Design review of the part built by this model. Coordinates are the model's own, in mm. A direction names the side the tool comes from. Coordinates: 2 decimals unless noted, no trailing zeros. Loops run counter-clockwise (first coordinate to the right, second up) from the corner with the lowest first, then second, coordinate; pieces in that order, holes last.
Q1. Draft analysis for pull direction Z (two halves, no side actions). For faces 6 (the face through (20.32, 58, 19)), 7 (the face through (0, -8, 38.1)), 8 (the face through (0, 58, 19.095)), 9 (the face through (6.846, 58, 23)), state which applies: released by +Z, released by -Z, zero draft, split by the parting line, or undercut.
Q2. Wall thickness on probe 1 along Y at (x, z) = (26.5, 2); probe 2 along X at (y, z) = (-6, 19.5); probe 3 along X at (y, z) = (19, 4.5): over which ranges is each line inside the solid? List them lowest first.
Q3. Add section B-B on x = 0. Give the number of separate pieces and of enclosed holes in the cut face, and give its area (3 significant figures).
Q4. Machinability: for faces 1 (the face through (0, -15.24, 28)), 2 (the face through (-0.674, -58.015, 27.798)), 3 (the face through (-7.733, 22, 6)), 4 (the face through (0, 66.04, 28)), 5 (the face through (20.32, -8, 19)), which of the approach directions +Z, -Z, +X, -X, +Y, -Y give a long, thin tool a straight path to every point of the face, cutting with its end or side? Answer none if there is none.
Q5. Add section A-A on y = 21.5. Give the boundary of the cut face in (x, z), and give its area (3 significant figures).
Q6. For P1, Ø4.5, axis at y = -9, z = 23, coming from the +X side; P2, Ø6, axis at y = 67.5, z = 21.5, coming from the -X side; P3, Ø7.5, axis at x = 3, z = 28.5, coming from the -Y side; P4, Ø14, axis at y = 57.5, z = 18.5, coming from the -X side, all flat-tipped, find the tip position at first contact; note any pin that passes through.
Q7. Add section C-C on z = 33.5. Give the boundary of the cut face in (x, y), and give its area (3 significant figures).
```python
from build123d import *

# Parameters (mm, degrees)
F1_DEPTH     = 12.7
F3_DEPTH     = 25.4
F4_R         = 12.7
F5_R         = 12.7
F6_R         = 12.7
F8_DEPTH     = 104.141
F9_W         = 26.8278098665
F9_H         = 37.2433126904
F10_DEPTH    = 12.701
F11_R        = 5.08
F12_R        = 12.1917967362
F12_R_2      = 5.1797647995
F13_DEPTH    = 5.08
F14_DEPTH    = 25.4
F15_SIZE     = 5.07999
F17_DEPTH    = 25.4
F18_R        = 5.08
F19_DEPTH    = 12.701
F21_DEPTH    = 12.701
F22_T1_DEPTH = 12.7
F23_R        = 2.794


# Not quite as in the source:
# - a fillet or chamfer that OpenCascade refuses, or shapes differently, is made with other operations: its cross-section is extruded or revolved along the edge and cut away or added
# - a fillet or chamfer is up to 0.001 mm smaller than in the source, because OpenCascade refuses the exact size
# - a feature names something its author has since deleted; it is built from what else it names


with BuildPart() as f1:
    # F0 (on Top) → F1 (new body)
    with BuildSketch(Plane.XY):
        Polygon((-50.8, 88.9), (-50.8, 0), (-50.8, -88.9), (0, -88.9), (50.8, -88.9), (50.8, 0), (50.8, 88.9), (0, 88.9), align=None)
    extrude(amount=F1_DEPTH)

    # F2 (on face) → F3 (join)
    with BuildSketch(Plane.XY.offset(12.7)):
        Polygon((20.32, 66.04), (0, 66.04), (-20.32, 66.04), (-20.32, 50.8), (0, 50.8), (20.32, 50.8), align=None)
        Polygon((0, 0), (-19.5459036618, 0), (-19.5459036618, -15.24), (0, -15.24), (20.32, -15.24), (20.32, 0), align=None)
    extrude(amount=F3_DEPTH)

    # F4
    f4_edges = [f1.edges().sort_by_distance(p)[0] for p in [
        (20.32, -7.62, 38.1),
        (-19.545904, -7.62, 38.1),
    ]]
    fillet(f4_edges, radius=F4_R)

    # F5
    f5_edges = [f1.edges().sort_by_distance(p)[0] for p in [
        (20.32, 58.42, 38.1),
        (-20.32, 58.42, 38.1),
    ]]
    fillet(f5_edges, radius=F5_R)

    # F6
    f6_edges = [f1.edges().sort_by_distance(p)[0] for p in [
        (50.8, 88.9, 6.35),
        (-50.8, 88.9, 6.35),
        (50.8, -88.9, 6.35),
        (-50.8, -88.9, 6.35),
    ]]
    fillet(f6_edges, radius=F6_R)

    # F7 (on face) → F8 (cut, through all)
    with BuildSketch(Plane.XZ.offset(15.24)):
        Polygon((6.8459036618, 27.6168659329), (0, 27.6168659329), (-6.8459036618, 27.6168659329), (-6.8459036618, 19.0950892866), (0, 19.0950892866), (6.8459036618, 19.0950892866), align=None)
    extrude(amount=-F8_DEPTH, mode=Mode.SUBTRACT)

    # F9 (on face) → F10 (cut, through all)
    with BuildSketch(Plane.XY.offset(12.7)):
        with Locations((-21.1466264445, 22.2513012122)):
            Rectangle(F9_W, F9_H)
        with Locations((21.1466264445, 22.2513012122)):
            Rectangle(F9_W, F9_H)
    extrude(amount=-F10_DEPTH, mode=Mode.SUBTRACT)

    # F11
    f11_edges = [f1.edges().sort_by_distance(p)[0] for p in [
        (-34.560531, 40.872958, 6.35),
        (-7.732722, 40.872958, 6.35),
        (-7.732722, 3.629645, 6.35),
        (-34.560531, 3.629645, 6.35),
        (34.560531, 3.629645, 6.35),
        (7.732722, 3.629645, 6.35),
        (7.732722, 40.872958, 6.35),
        (34.560531, 40.872958, 6.35),
    ]]
    fillet(f11_edges, radius=F11_R)

    # F12 (on face) → F13 (join)
    with BuildSketch(Plane.XY.offset(12.7)):
        with Locations((0, -63.150562346)):
            Circle(F12_R)
        with Locations((0, -63.150562346)):
            Circle(F12_R_2, mode=Mode.SUBTRACT)
    extrude(amount=F13_DEPTH)

    # F14 (add): a face of the model
    f14_faces = [f1.faces().sort_by_distance(p)[0] for p in [
        (0, -63.150562346, 12.7),
    ]]
    extrude(f14_faces, amount=F14_DEPTH)

    # F15 (size 5.08 in the source; OpenCascade refuses exactly that, so slightly less here)
    f15_edges = [f1.edges().sort_by_distance(p)[0] for p in [
        (-12.191797, -63.150562, 17.78),
    ]]
    chamfer(f15_edges, length=F15_SIZE)

    # F16 (on face) → F17 (cut)
    with BuildSketch(Plane.XY.offset(12.7)):
        with BuildLine():
            Line((-9.2206190628, -29.6420995146), (-33.0726338262, -29.6420995146))
            Line((-33.0726338262, -29.6420995146), (-33.0726338262, -61.3056821097))
            Line((-33.0726338262, -61.3056821097), (-20.1783736468, -61.3056821097))
            ThreePointArc((-20.1783736468, -61.3056821097), (-16.7830306246, -51.7971386698), (-9.2206190628, -45.1075434685))
            Line((-9.2206190628, -45.1075434685), (-9.2206190628, -29.6420995146))
        make_face()
        with BuildLine():
            Line((33.0726338262, -29.6420995146), (9.2206190628, -29.6420995146))
            Line((9.2206190628, -29.6420995146), (9.2206190628, -45.1075434685))
            ThreePointArc((9.2206190628, -45.1075434685), (16.7830306246, -51.7971386698), (20.1783736468, -61.3056821097))
            Line((20.1783736468, -61.3056821097), (33.0726338262, -61.3056821097))
            Line((33.0726338262, -61.3056821097), (33.0726338262, -29.6420995146))
        make_face()
    extrude(amount=-F17_DEPTH, mode=Mode.SUBTRACT)

    # F18
    f18_edges = [f1.edges().sort_by_distance(p)[0] for p in [
        (-9.220619, -29.6421, 6.35),
        (-33.072634, -29.6421, 6.35),
        (-33.072634, -61.305682, 6.35),
        (33.072634, -61.305682, 6.35),
        (33.072634, -29.6421, 6.35),
        (9.220619, -29.6421, 6.35),
    ]]
    fillet(f18_edges, radius=F18_R)

    # F16 (on face) → F19 (cut, through all)
    with BuildSketch(Plane.XY.offset(12.7)):
        with BuildLine():
            Line((-9.2206190628, -29.6420995146), (-33.0726338262, -29.6420995146))
            Line((-33.0726338262, -29.6420995146), (-33.0726338262, -61.3056821097))
            Line((-33.0726338262, -61.3056821097), (-20.1783736468, -61.3056821097))
            ThreePointArc((-20.1783736468, -61.3056821097), (-16.7830306246, -51.7971386698), (-9.2206190628, -45.1075434685))
            Line((-9.2206190628, -45.1075434685), (-9.2206190628, -29.6420995146))
        make_face()
        with BuildLine():
            Line((33.0726338262, -29.6420995146), (9.2206190628, -29.6420995146))
            Line((9.2206190628, -29.6420995146), (9.2206190628, -45.1075434685))
            ThreePointArc((9.2206190628, -45.1075434685), (16.7830306246, -51.7971386698), (20.1783736468, -61.3056821097))
            Line((20.1783736468, -61.3056821097), (33.0726338262, -61.3056821097))
            Line((33.0726338262, -61.3056821097), (33.0726338262, -29.6420995146))
        make_face()
    extrude(amount=-F19_DEPTH, mode=Mode.SUBTRACT)

    # F20 (on face) → F21 (cut, through all)
    with BuildSketch(Plane.XY.offset(12.7)):
        with BuildLine():
            Line((-33.0726338262, -81.930026412), (-9.2206190628, -81.930026412))
            ThreePointArc((-9.2206190628, -81.930026412), (-14.9601496341, -77.7752677938), (-18.9837029569, -71.9430084535))
            Line((-18.9837029569, -71.9430084535), (-33.0726338262, -71.9430084535))
            Line((-33.0726338262, -71.9430084535), (-33.0726338262, -81.930026412))
        make_face()
        with BuildLine():
            ThreePointArc((18.9837029569, -71.9430084535), (14.9601496341, -77.7752677938), (9.2206190628, -81.930026412))
            Line((9.2206190628, -81.930026412), (33.0726338262, -81.930026412))
            Line((33.0726338262, -81.930026412), (33.0726338262, -71.9430084535))
            Line((33.0726338262, -71.9430084535), (18.9837029569, -71.9430084535))
        make_face()
    extrude(amount=-F21_DEPTH, mode=Mode.SUBTRACT)

    # F22: fillet of radius 5.08 on 10 edges, made by hand

    # F22_s2 → F22_t1 (join)
    with BuildSketch(Plane.XY):
        with BuildLine():
            ThreePointArc((-9.2206190628, -34.7220995146), (-10.7085166144, -31.1299970662), (-14.3006190628, -29.6420995146))
            Line((-14.3006190628, -29.6420995146), (-9.2206190628, -29.6420995146))
            Line((-9.2206190628, -29.6420995146), (-9.2206190628, -34.7220995146))
        make_face()
        with BuildLine():
            ThreePointArc((-27.9926338262, -29.6420995146), (-31.5847362746, -31.1299970662), (-33.0726338262, -34.7220995146))
            Line((-33.0726338262, -34.7220995146), (-33.0726338262, -29.6420995146))
            Line((-33.0726338262, -29.6420995146), (-27.9926338262, -29.6420995146))
        make_face()
        with BuildLine():
            ThreePointArc((-33.0726338262, -56.2256821097), (-31.5847362746, -59.8177845582), (-27.9926338262, -61.3056821097))
            Line((-27.9926338262, -61.3056821097), (-33.0726338262, -61.3056821097))
            Line((-33.0726338262, -61.3056821097), (-33.0726338262, -56.2256821097))
        make_face()
        with BuildLine():
            ThreePointArc((33.0726338262, -34.7220995146), (31.5847362746, -31.1299970662), (27.9926338262, -29.6420995146))
            Line((27.9926338262, -29.6420995146), (33.0726338262, -29.6420995146))
            Line((33.0726338262, -29.6420995146), (33.0726338262, -34.7220995146))
        make_face()
        with BuildLine():
            ThreePointArc((14.3006190628, -29.6420995146), (10.7085166144, -31.1299970662), (9.2206190628, -34.7220995146))
            Line((9.2206190628, -34.7220995146), (9.2206190628, -29.6420995146))
            Line((9.2206190628, -29.6420995146), (14.3006190628, -29.6420995146))
        make_face()
        with BuildLine():
            ThreePointArc((27.9926338262, -61.3056821097), (31.5847362746, -59.8177845582), (33.0726338262, -56.2256821097))
            Line((33.0726338262, -56.2256821097), (33.0726338262, -61.3056821097))
            Line((33.0726338262, -61.3056821097), (27.9926338262, -61.3056821097))
        make_face()
        with BuildLine():
            ThreePointArc((-33.0726338262, -76.850026412), (-31.5847362746, -80.4421288604), (-27.9926338262, -81.930026412))
            Line((-27.9926338262, -81.930026412), (-33.0726338262, -81.930026412))
            Line((-33.0726338262, -81.930026412), (-33.0726338262, -76.850026412))
        make_face()
        with BuildLine():
            ThreePointArc((-27.9926338262, -71.9430084535), (-31.5847362746, -73.4309060051), (-33.0726338262, -77.0230084535))
            Line((-33.0726338262, -77.0230084535), (-33.0726338262, -71.9430084535))
            Line((-33.0726338262, -71.9430084535), (-27.9926338262, -71.9430084535))
        make_face()
        with BuildLine():
            ThreePointArc((33.0726338262, -77.0230084535), (31.5847362746, -73.4309060051), (27.9926338262, -71.9430084535))
            Line((27.9926338262, -71.9430084535), (33.0726338262, -71.9430084535))
            Line((33.0726338262, -71.9430084535), (33.0726338262, -77.0230084535))
        make_face()
        with BuildLine():
            ThreePointArc((27.9926338262, -81.930026412), (31.5847362746, -80.4421288604), (33.0726338262, -76.850026412))
            Line((33.0726338262, -76.850026412), (33.0726338262, -81.930026412))
            Line((33.0726338262, -81.930026412), (27.9926338262, -81.930026412))
        make_face()
    extrude(amount=F22_T1_DEPTH)

    # F23
    f23_edges = [f1.edges().sort_by_distance(p)[0] for p in [
        (9.220619, -81.930026, 6.35),
        (-9.220619, -81.930026, 6.35),
    ]]
    fillet(f23_edges, radius=F23_R)


solid = f1.part
```
Entries:
1. face 6: zero draft
1. face 7: released by +Z
1. face 8: undercut
1. face 9: undercut
2. probe 1: y = -88.9 to -81.93, -71.94 to -61.31, -29.64 to 3.63, 40.87 to 88.9
2. probe 2: x = -19.55 to -6.85, 6.85 to 20.32
2. probe 3: x = -50.8 to -34.56, -7.73 to 7.73, 34.56 to 50.8
3. separate pieces: 3
3. enclosed holes: 0
3. area: 3,080 mm2
4. face 1: +Z, +X, -X
4. face 2: +Z
4. face 3: +Z, -Z
4. face 4: +Z, +X, -X, +Y
4. face 5: +Z, +X, +Y, -Y
5. outline: (-50.8, 0) - (-34.56, 0) - (-34.56, 12.7) - (-50.8, 12.7) - close; (-7.73, 0) - (7.73, 0) - (7.73, 12.7) - (-7.73, 12.7) - close; (34.56, 0) - (50.8, 0) - (50.8, 12.7) - (34.56, 12.7) - close
5. area: 609 mm2
6. P1: stops at x = 20.32
6. P2: stops at x = -20.32
6. P3: stops at y = -68.33
6. P4: stops at x = -50.8
7. outline: (-17.4, 50.8) - (17.4, 50.8) - (17.4, 66.04) - (-17.4, 66.04) - close; (-16.63, -15.24) - (17.4, -15.24) - (17.4, 0) - (-16.63, 0) - close; circle Ø10.36 at (0, -63.15)
7. area: 1,130 mm2
